Here's how the part is built. I have some questions about the finished solid (model axes, mm). A direction names the side the tool comes from. Round coordinates to 2 decimals unless told otherwise and drop trailing zeros. Use one line per item in the form item = value. Start each with the question number.
Item 1: I'm going to push flat-ended pins straight in: pin 1 Ø12 at (x, z) = (-7.5, -1) entering from -Y; pin 2 Ø1.5 at (x, y) = (5, 7) entering from +Z; pin 3 Ø3 at (x, y) = (-5, -4) entering from -Z; pin 4 Ø10 at (x, y) = (-8.5, 5) entering from -Z. Where does each tip first touch, or does it pass through?
Item 2: Thinking about a two-plate mould opening in X: for faces 4 (the face through (0, 3, -3)), 5 (the face through (-6, 9.5, 6)), which applies, released by +X, released by -X, zero draft, split by the parting line, or undercut?
Item 3: If I drill on L1, parallel to Z at x = 0, y = -3.3; L2, parallel to Z at x = 0, y = 4.9; L3, parallel to X at y = -3.25, z = 0, over which ranges is the centre line in solid material (lowest first)? Write a range as [from, to].
Item 4: If we section it at A-A (y = -2.5): State how many separate pieces and enclosed holes the cut face has, then the cut area to 3 significant figures.
Item 5: For faces 1 (the face through (5.96, 5.22, 1.88)), 2 (the face through (-1.73, -2.19, -7.81)), 3 (the face through (-0.54, -3.29, -2.44)), which set-ups out of +Z, -Z, +X, -X, +Y, -Y let a thin tool reach every point of the face, with its end or its side?
```python
from build123d import *

# Parameters (mm, degrees)
F0_R          = 8
F0_R_2        = 6.25
F4_DEPTH      = 25
F0_R_3        = 2.5
F5_DEPTH      = 20
F5_DEPTH_BACK = 4
F6_START      = -3
F6_DEPTH      = 6.5005844247
F1_W          = 6
F1_H          = 1
F7_DEPTH      = 25
F8_R          = 2


with BuildPart() as f3:
    # F2 (on Right) → F3 (revolve)
    with BuildSketch(Plane.YZ):
        with BuildLine():
            Line((9.4995843247, 0), (9.4995843247, 10.2535216138))
            ThreePointArc((9.4995843247, 10.2535216138), (-2.6924670032, 9.0038209902), (-11.0074579716, 0))
            Line((-11.0074579716, 0), (9.4995843247, 0))
        make_face()
    revolve(axis=Axis((0, -0.7539368235, 0), (0, -1, 0)))

    # F0 (on Front) → F4 (cut)
    with BuildSketch(Plane.XZ):
        Circle(F0_R)
        Circle(F0_R_2, mode=Mode.SUBTRACT)
    extrude(amount=F4_DEPTH, mode=Mode.SUBTRACT)

    # F0 (on Front) → F5 (cut, two sides)
    with BuildSketch(Plane.XZ) as f5_sk:
        Circle(F0_R_3)
    extrude(amount=F5_DEPTH, mode=Mode.SUBTRACT)
    extrude(f5_sk.sketch, amount=-F5_DEPTH_BACK, mode=Mode.SUBTRACT)

    # F0 (on Front) → F6 (cut)
    with BuildSketch(Plane.XZ.offset(F6_START)):
        Circle(F0_R_2)
        Circle(F0_R_3, mode=Mode.SUBTRACT)
        Circle(F0_R_3)
    extrude(amount=-F6_DEPTH, mode=Mode.SUBTRACT)

    # F1 (on Front) → F7 (cut)
    with BuildSketch(Plane.XZ):
        with Locations((-4, 0.0314258505)):
            Rectangle(F1_W, F1_H)
        Polygon((0.0397717133, -1.131738329), (3.0397717133, -6.3278907517), (3.9057971171, -5.8278907517), (0.9057971171, -0.631738329), align=None)
        Polygon((0.9602282867, 0.6003124786), (3.9602282867, 5.7964649013), (3.0942028829, 6.2964649013), (0.0942028829, 1.1003124786), align=None)
    extrude(amount=F7_DEPTH, mode=Mode.SUBTRACT)

    # F8
    f8_edges = [f3.edges().sort_by_distance(p)[0] for p in [
        (0, 9.499584, -10.253522),
        (-6.25, 9.499584, 0),
    ]]
    fillet(f8_edges, radius=F8_R)


solid = f3.part
```
Values found:
q1.pin_1 = -9.75
q1.pin_2 = 9.86
q1.pin_3 = -7.96
q1.pin_4 = -10.25
q2.face_4 = undercut
q2.face_5 = zero draft
q3.L1 = [-8.68, -8], [-6.25, -2.5], [2.5, 6.25], [8, 8.68]
q3.L2 = [-10.83, -6.25], [6.25, 10.83]
q3.L3 = [-8.71, -8], [2.5, 6.25], [8, 8.71]
q4.separate_pieces = 4
q4.enclosed_holes = 1
q4.area = 151 mm2
q5.face_1 = +Y
q5.face_2 = -Y
q5.face_3 = +Y, -Y
